The listing builds one solid part. Answer for the finished solid, in the listing's coordinates (mm). A direction names the side the tool comes from. Round coordinates to 2 decimals unless told otherwise and drop trailing zeros. Write each loop counter-clockwise with the first axis right and the second up, starting at its lowest first coordinate (ties: lowest second). Pieces come first, ordered by that corner, then holes.
(1) For faces 1 (the face through (-40, 1, 0)), 2 (the face through (-23, 2, -6)), determine the directions among +Z, -Z, +X, -X, +Y, -Y from which every point of the face is accessible in a straight line to the end or side of a thin tool.
(2) A cutting plane is placed at B-B, the plane z = 0. Give the vertices of the cut face in (x, y).
(3) A cutting plane is placed at A-A, the plane x = -8.85. Give the vertices of the cut face in (y, z).
(4) The mould has two halves that part along Z. Classify faces 3 (the face through (8, 3, 0)), 4 (the face through (-34, 2, 0)), 5 (the face through (-1, 1, 8)): +Z half, -Z half, draft (parallel to the pull), parting line (faces both ways), or undercut.
(5) A cutting plane is placed at D-D, the plane x = -21.5. Give the vertices of the cut face in (y, z), and give its area (3 significant figures).
(6) Find the intervals of material crossed by probe 1 along X at (y, z) = (1.05, 0); probe 2 along X at (y, z) = (2.15, -1.75); probe 3 along X at (y, z) = (0.75, 1), in increasing order.
(7) A cutting plane is placed at C-C, the plane y = 0.7. Give the vertices of the cut face in (x, z).
from build123d import *

# Parameters (mm, degrees)
SKETCH1_W           = 80
SKETCH1_H           = 16
BOSS_EXTRUDE1_DEPTH = 3
SKETCH2_R           = 1.2
SKETCH2_W           = 23
SKETCH2_H           = 12
CUT_EXTRUDE1_DEPTH  = 4


with BuildPart() as part:
    # Sketch1 → Boss-Extrude1 (new body)
    with BuildSketch(Plane(origin=(0, 0, 0), x_dir=(1, 0, 0), z_dir=(0, 1, 0))):
        Rectangle(SKETCH1_W, SKETCH1_H)
    extrude(amount=BOSS_EXTRUDE1_DEPTH)

    # Sketch2 → Cut-Extrude1 (cut, through all)
    with BuildSketch(Plane(origin=(0, 3, 0), x_dir=(1, 0, 0), z_dir=(0, 1, 0))):
        with Locations((-36.15, 0)):
            Circle(SKETCH2_R)
        with Locations((-8.85, 0)):
            Circle(SKETCH2_R)
        with Locations((-22.5, 0)):
            Rectangle(SKETCH2_W, SKETCH2_H)
    extrude(amount=-CUT_EXTRUDE1_DEPTH, mode=Mode.SUBTRACT)


solid = part.part
Solutions:
1. face 1: +Z, -Z, -X, +Y, -Y
1. face 2: +Y, -Y
2. outline: (-40, 0) - (-37.35, 0) - (-37.35, 3) - (-40, 3) - close; (-34.95, 0) - (-34, 0) - (-34, 3) - (-34.95, 3) - close; (-11, 0) - (-10.05, 0) - (-10.05, 3) - (-11, 3) - close; (-7.65, 0) - (40, 0) - (40, 3) - (-7.65, 3) - close
3. outline: (0, -8) - (3, -8) - (3, -1.2) - (0, -1.2) - close; (0, 1.2) - (3, 1.2) - (3, 8) - (0, 8) - close
4. face 3: draft
4. face 4: undercut
4. face 5: +Z half
5. outline: (0, -8) - (3, -8) - (3, -6) - (0, -6) - close; (0, 6) - (3, 6) - (3, 8) - (0, 8) - close
5. area: 12.0 mm2
6. probe 1: x = -40 to -37.35, -34.95 to -34, -11 to -10.05, -7.65 to 40
6. probe 2: x = -40 to -34, -11 to 40
6. probe 3: x = -40 to -36.81, -35.49 to -34, -11 to -9.51, -8.19 to 40
7. outline: (-40, -8) - (40, -8) - (40, 8) - (-40, 8) - close; hole circle Ø2.4 at (-36.15, 0); hole (-34, -6) - (-11, -6) - (-11, 6) - (-34, 6) - close; hole circle Ø2.4 at (-8.85, 0)
